Geometry: see drawing. Coordinates: mm, zero at the bounding-box minimum. A direction names the side the tool comes from. Coordinates: 2 decimals unless noted, no trailing zeros. Order: outer loops, then holes, each group sorted by start corner. A loop starts at its lowest first (then second) coordinate and runs counter-clockwise, first axis right, second up.
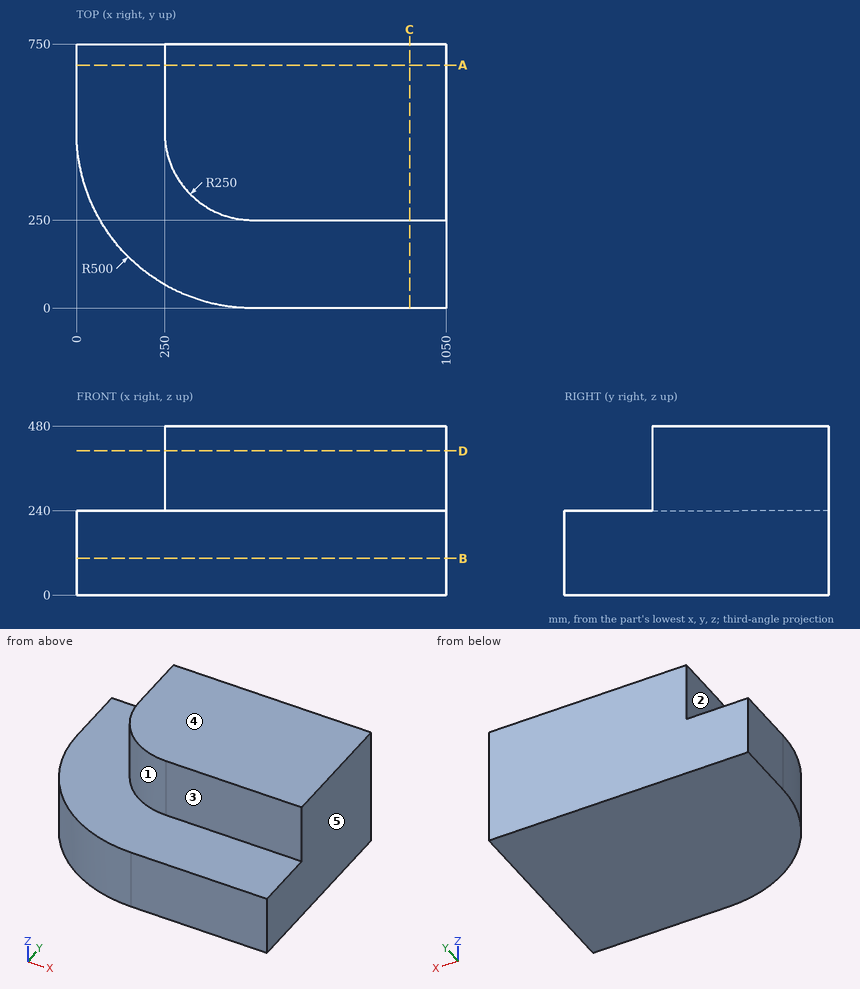
Item 1: Access query for the marked faces 1, 2, 3, 4 and 5. Directions: +Z, -Z, +X, -X, +Y, -Y. A direction counts if a zero-diameter tool reaches every point of the face in a straight line with its end or side. Return the directions, or none.
Response values:
face 1: +Z, -X, -Y
face 2: +Z, -X, +Y, -Y
face 3: +Z, +X, -X, -Y
face 4: +Z, +X, -X, +Y, -Y
face 5: +Z, -Z, +X, +Y, -Y
Item 2: Cut plane C-C on x = 945.5. Return loops of the section in (y, z).
Response values:
outline: (0, 0) - (750, 0) - (750, 480) - (250, 480) - (250, 240) - (0, 240) - close
Item 3: Cut plane D-D on z = 409.5. Return loops of the section in (x, y).
Response values:
outline: (250, 500) arc R250 ccw to (500, 250) - (1050, 250) - (1050, 750) - (250, 750) - close
Item 4: Pin query (flat end, axial travel): pin 1 Ø1 at (x, y) = (113, 415) entering from +Z; pin 2 Ø5 at (y, z) = (561, 330.5) entering from -X; pin 3 Ø5 at (x, z) = (577, 55) entering from -Y. Return the tip coordinate at first contact, or that it passes through.
Response values:
pin 1: stops at z = 240
pin 2: stops at x = 250
pin 3: stops at y = 0
Item 5: Ray query, probe 1 along Y at (x, z) = (851, 307.5); probe 2 along Z at (x, y) = (952, 48); probe 3 along Y at (x, z) = (489, 254.5). Return the intervals inside material, ascending.
Response values:
probe 1: y = 250 to 750
probe 2: z = 0 to 240
probe 3: y = 250.24 to 750
Item 6: Cut plane B-B on z = 104.5. Return loops of the section in (x, y), then the cut area to 3 significant figures.
Response values:
outline: (0, 500) arc R500 ccw to (500, 0) - (1050, 0) - (1050, 750) - (0, 750) - close
area: 734,000 mm2
Item 7: Cut plane A-A on y = 690. Return loops of the section in (x, z), then the cut area to 3 significant figures.
Response values:
outline: (0, 0) - (1050, 0) - (1050, 480) - (250, 480) - (250, 240) - (0, 240) - close
area: 444,000 mm2
